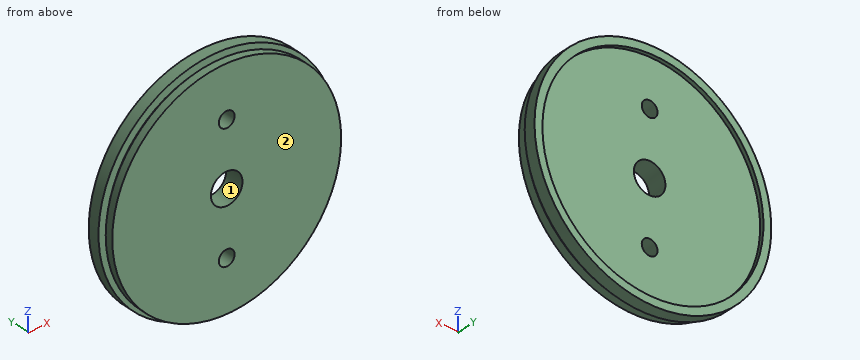
Autodesk Inventor part; units mm, degrees
ref_plane "YZ Plane" through (0, 0, 0) normal (1, 0, 0) x (0, 1, 0)
ref_plane "XZ Plane" through (0, 0, 0) normal (0, 1, 0) x (-1, 0, 0)
ref_plane "XY Plane" through (0, 0, 0) normal (0, 0, 1) x (1, 0, 0)
sketch "Sketch1" plane through (0, 0, 0) normal (0, 1, 0) x (-1, 0, 0)
  circle A0 centre (0, 0) radius 92.075
  dimension "d0" = 184.15
extrude "Extrusion1" add sketch "Sketch1" along normal blind 6.35
sketch "Sketch2" plane through (0, 6.35, 0) normal (0, 1, 0) x (1, 0, 0)
  circle A0 centre (0, 0) radius 88.9
  dimension "d3" = 177.8
extrude "Extrusion2" add sketch "Sketch2" along normal blind 3.175
sketch "Sketch3" plane through (0, 9.525, 0) normal (0, 1, 0) x (1, 0, 0)
  circle A0 centre (0, 0) radius 95.25
  dimension "d6" = 190.5
extrude "Extrusion3" add sketch "Sketch3" along normal blind 6.35
sketch "Sketch8" plane through (0, 15.875, 0) normal (0, 1, 0) x (1, 0, 0)
  circle A0 centre (0, 0) radius 95.25
  circle A1 centre (0, 0) radius 88.9
  dimension "d33" = 177.8
  dimension "d34" = 190.5
extrude "Extrusion9" add sketch "Sketch8" along normal blind 3.175
sketch "Sketch9" plane through (0, 15.875, 0) normal (0, 1, 0) x (1, 0, 0)
  circle A0 centre (0, 0) radius 12.7
  circle A1 centre (0, -50.8) radius 6.35
  circle A2 centre (0, 50.8) radius 6.35
  dimension "d37" = 12.7
  dimension "d38" = 50.8
  dimension "d39" = 50.8
  dimension "d40" = 25.4
extrude "Extrusion10" cut sketch "Sketch9" against normal through all
properties part number "upper_thermal_barrier" material "Phenolic Resin"
For this review, take the finished solid that the model builds, in its own axes (mm). Face numbers are marked on the shaded views. Round coordinates to 2 decimals unless told otherwise and drop trailing zeros. Write each loop counter-clockwise with the first axis right and the second up, starting at its lowest first coordinate (ties: lowest second). Pieces come first, ordered by that corner, then holes. Notation, with made-up numbers: (71.25, 49) - (81.25, 49) arc R20 ccw to (81.25, 69) - close; hole circle Ø8 at (-25.5, -18.75). An arc over 180 degrees is marked (long way). Use CSV: the item, a comma, the result in double quotes.
1) Add section D-D on z = -53.5. Write out the cut boundary in (x, y) (3 decimals), and give its area (3 significant figures).
Conclusion:
outline,"(-78.806, 9.525) - (-71, 9.525) - (-71, 6.35) - (-74.937, 6.35) - (-74.937, 0) - (-5.747, 0) - (-5.747, 15.875) - (-71, 15.875) - (-71, 19.05) - (-78.806, 19.05) - close; (5.747, 0) - (74.937, 0) - (74.937, 6.35) - (71, 6.35) - (71, 9.525) - (78.806, 9.525) - (78.806, 19.05) - (71, 19.05) - (71, 15.875) - (5.747, 15.875) - close"
area,"2,270 mm^2"
2) Add section A-A on x = 0. Write out the cut boundary in (y, z) (3 decimals).
Conclusion:
outline,"(0, -92.075) - (6.35, -92.075) - (6.35, -88.9) - (9.525, -88.9) - (9.525, -95.25) - (19.05, -95.25) - (19.05, -88.9) - (15.875, -88.9) - (15.875, -57.15) - (0, -57.15) - close; (0, -44.45) - (15.875, -44.45) - (15.875, -12.7) - (0, -12.7) - close; (0, 12.7) - (15.875, 12.7) - (15.875, 44.45) - (0, 44.45) - close; (0, 57.15) - (15.875, 57.15) - (15.875, 88.9) - (19.05, 88.9) - (19.05, 95.25) - (9.525, 95.25) - (9.525, 88.9) - (6.35, 88.9) - (6.35, 92.075) - (0, 92.075) - close"
3) Add section B-B on z = 0. Write out the cut boundary in (x, y) (3 decimals), and give its area (3 significant figures).
Conclusion:
outline,"(-95.25, 9.525) - (-88.9, 9.525) - (-88.9, 6.35) - (-92.075, 6.35) - (-92.075, 0) - (-12.7, 0) - (-12.7, 15.875) - (-88.9, 15.875) - (-88.9, 19.05) - (-95.25, 19.05) - close; (12.7, 0) - (92.075, 0) - (92.075, 6.35) - (88.9, 6.35) - (88.9, 9.525) - (95.25, 9.525) - (95.25, 19.05) - (88.9, 19.05) - (88.9, 15.875) - (12.7, 15.875) - close"
area,"2,580 mm^2"
4) Wall thickness on line 1 along Z through (x, y) = (0, 6.25) (3 decimals); line 2 along Z through (x, y) = (0, 11.25); line 3 along Z through (x, y) = (0, 17.15): over which ranges is each line inside the solid? List them lowest first. Write a range as from..to.
Conclusion:
line 1,"z = -92.075..-57.15, -44.45..-12.7, 12.7..44.45, 57.15..92.075"
line 2,"z = -95.25..-57.15, -44.45..-12.7, 12.7..44.45, 57.15..95.25"
line 3,"z = -95.25..-88.9, 88.9..95.25"
5) The part is to be moulded in two halves that separate along X. For the marked faces 1 and 2, say which applies: pulls with the +X half, pulls with the -X half, needs draft (parallel to the pull), parting line crosses it, or undercut.
Conclusion:
face 1,"undercut"
face 2,"needs draft"
6) Add section C-C on z = 25. Write out the cut boundary in (x, y) (3 decimals), and give its area (3 significant figures).
Conclusion:
outline,"(-91.911, 9.525) - (-85.312, 9.525) - (-85.312, 6.35) - (-88.616, 6.35) - (-88.616, 0) - (88.616, 0) - (88.616, 6.35) - (85.312, 6.35) - (85.312, 9.525) - (91.911, 9.525) - (91.911, 19.05) - (85.312, 19.05) - (85.312, 15.875) - (-85.312, 15.875) - (-85.312, 19.05) - (-91.911, 19.05) - close"
area,"2,880 mm^2"
7) Clearance check with flat-ended pins moving along their axes: pin 1 Ø2 at (x, z) = (50, 41) entering from -Y; pin 2 Ø14.5 at (x, z) = (0, -50.8) entering from +Y (3 decimals); pin 3 Ø2 at (y, z) = (10.5, 27.5) entering from -X; pin 4 Ø6 at (y, z) = (6, -8) entering from +X. State where each tip first meets the part, or that it passes through.
Conclusion:
pin 1,"stops at y = 0"
pin 2,"stops at y = 15.875"
pin 3,"stops at x = -91.49"
pin 4,"stops at x = 91.94"
